Here's how the part is built. I have some questions about the finished solid (model axes, mm). Give positions to 0.01 mm unless a question says otherwise; leave off trailing zeros. Loops run counter-clockwise (first coordinate to the right, second up) from the corner with the lowest first, then second, coordinate; pieces in that order, holes last. Notation, with made-up numbers: M 51.25,6 L 107.25,6 A14 ccw 107.25,17 Z; hole C 64.25,29.25 d3. An arc over 180 degrees is marked long. Answer as CSV lines item,"result". Start each with the question number.
Item 1: I want a section at A-A on y = -57.95. List the corners of the cut face in (x, z) for me, plus the area to 3 significant figures.
Item 2: I want a section at B-B on x = 0. List the corners of the cut face in (y, z) for me.
Item 3: If I drill on line 1 along Y through (x, z) = (-72.95, 12.25); line 2 along Y through (x, z) = (0, 12.5), over which ranges is the centre line in solid material (lowest first)? Write a range as from..to.
Item 4: If we mould it in two halves opening along Y, with no side actions, what happens to faces 1 (the cylindrical face through (-105.811, 105.695, 12.878)), 2 (the flat face through (-2, 26, 25.4)), 3 (the cylindrical face through (-74.565, -61.055, 12.522))? For each: released by +Y, released by -Y, zero draft, split by the parting line, or undercut.
Item 5: Will this pin go through, and if not, where does the flat tip stop? P1, Ø4, axis at x = 10.5, y = 70.5, coming from the -Z side.
from build123d import *

# Parameters (mm, degrees)
F0_W     = 215.9
F0_H     = 215.9
F1_DEPTH = 25.4
F3_D     = 10.8
F4_R     = 7.5
F6_D     = 7


with BuildPart() as f1:
    # F0 (on Top) → F1 (new body)
    with BuildSketch(Plane.XY):
        Rectangle(F0_W, F0_H)
    extrude(amount=F1_DEPTH)

    # F3 (through all)
    with Locations(Plane.XY.offset(25.4)):
        with Locations((0, 0)):
            Hole(F3_D / 2)

    # F4
    f4_edges = [f1.edges().sort_by_distance(p)[0] for p in [
        (-107.95, -107.95, 12.7),
        (107.95, -107.95, 12.7),
        (107.95, 107.95, 12.7),
        (-107.95, 107.95, 12.7),
    ]]
    fillet(f4_edges, radius=F4_R)

    # F6 (through all)
    with Locations(Plane.XY.offset(25.4)):
        with Locations((-72.95, -57.95)):
            Hole(F6_D / 2)


solid = f1.part
Result:
1,outline,"M -107.95,0 L -76.45,0 L -76.45,25.4 L -107.95,25.4 Z; M -69.45,0 L 107.95,0 L 107.95,25.4 L -69.45,25.4 Z"
1,area,"5,310 mm^2"
2,outline,"M -107.95,0 L -5.4,0 L -5.4,25.4 L -107.95,25.4 Z; M 5.4,0 L 107.95,0 L 107.95,25.4 L 5.4,25.4 Z"
3,line 1,"-107.95..-61.45, -54.45..107.95"
3,line 2,"-107.95..-5.4, 5.4..107.95"
4,face 1,"released by +Y"
4,face 2,"zero draft"
4,face 3,"undercut"
5,P1,"z = 0"
